from build123d import *

# Parameters (mm, degrees)
ESQUISSE1_W        = 383
ESQUISSE1_H        = 30
BOSS_EXTRU_1_DEPTH = 10
ESQUISSE2_W        = 10
ESQUISSE2_H        = 30
BOSS_EXTRU_2_DEPTH = 20
ESQUISSE3_W        = 10
ESQUISSE3_H        = 100
BOSS_EXTRU_3_DEPTH = 5


with BuildPart() as part:
    # Esquisse1 → Boss.-Extru.1 (new body)
    with BuildSketch(Plane.XY):
        Rectangle(ESQUISSE1_W, ESQUISSE1_H)
    extrude(amount=BOSS_EXTRU_1_DEPTH)

    # Esquisse2 → Boss.-Extru.2 (add)
    with BuildSketch(Plane.XY.offset(10)):
        with Locations((-186.5, 0)):
            Rectangle(ESQUISSE2_W, ESQUISSE2_H)
        with Locations((-166.5, 0)):
            Rectangle(ESQUISSE2_W, ESQUISSE2_H)
        with Locations((-146.5, 0)):
            Rectangle(ESQUISSE2_W, ESQUISSE2_H)
        with Locations((-126.5, 0)):
            Rectangle(ESQUISSE2_W, ESQUISSE2_H)
        with Locations((-106.5, 0)):
            Rectangle(ESQUISSE2_W, ESQUISSE2_H)
        with Locations((-86.5, 0)):
            Rectangle(ESQUISSE2_W, ESQUISSE2_H)
        with Locations((-66.5, 0)):
            Rectangle(ESQUISSE2_W, ESQUISSE2_H)
        with Locations((-46.5, 0)):
            Rectangle(ESQUISSE2_W, ESQUISSE2_H)
        with Locations((-26.5, 0)):
            Rectangle(ESQUISSE2_W, ESQUISSE2_H)
        with Locations((-6.5, 0)):
            Rectangle(ESQUISSE2_W, ESQUISSE2_H)
        with Locations((13.5, 0)):
            Rectangle(ESQUISSE2_W, ESQUISSE2_H)
        with Locations((33.5, 0)):
            Rectangle(ESQUISSE2_W, ESQUISSE2_H)
        with Locations((53.5, 0)):
            Rectangle(ESQUISSE2_W, ESQUISSE2_H)
        with Locations((73.5, 0)):
            Rectangle(ESQUISSE2_W, ESQUISSE2_H)
        with Locations((93.5, 0)):
            Rectangle(ESQUISSE2_W, ESQUISSE2_H)
        with Locations((113.5, 0)):
            Rectangle(ESQUISSE2_W, ESQUISSE2_H)
        with Locations((133.5, 0)):
            Rectangle(ESQUISSE2_W, ESQUISSE2_H)
        with Locations((153.5, 0)):
            Rectangle(ESQUISSE2_W, ESQUISSE2_H)
        Polygon((168.5, -15), (178.5, -15), (191.5, -15), (191.5, 15), (178.5, 15), (168.5, 15), align=None)
    extrude(amount=BOSS_EXTRU_2_DEPTH)

    # Esquisse3 → Boss.-Extru.3 (add)
    with BuildSketch(Plane.XZ.offset(15)):
        with Locations((0, -41.837008413)):
            Rectangle(ESQUISSE3_W, ESQUISSE3_H)
    extrude(amount=BOSS_EXTRU_3_DEPTH)


solid = part.part
Model file for the job. Use its own axes, mm. A direction names the side the tool comes from. Give positions to 0.01 mm unless a question says otherwise; leave off trailing zeros. Loops run counter-clockwise (first coordinate to the right, second up) from the corner with the lowest first, then second, coordinate; pieces in that order, holes last.
Item 1: Slice it at B-B (z = -7). Write the cut outline in (x, y), plus the area to 3 significant figures.
Check values:
outline: (-5, -20) - (5, -20) - (5, -15) - (-5, -15) - close
area: 50.0 mm2
Item 2: Drop flat-ended pins along their axis: P1, Ø4, axis at y = -13.5, z = -29, coming from the +X side; P2, Ø24, axis at x = -36.5, z = 20, coming from the -Y side; P3, Ø2, axis at x = -4, y = 7.5, coming from the -Z side; P4, Ø1, axis at x = -144, z = -2, coming from the +Y side. Give the stop position or say it passes through.
Check values:
P1: stops at x = 5
P2: stops at y = -15
P3: stops at z = 0
P4: passes through
Item 3: Drill centre lines: line 1 along Z through (x, y) = (-59, 4); line 2 along Z through (x, y) = (-29, -8); line 3 along X through (y, z) = (-17.5, -20). Where is each one in solid material? Low to high.
Check values:
line 1: z = 0 to 10
line 2: z = 0 to 30
line 3: x = -5 to 5
Item 4: Which spindle directions (+Z, -Z, +X, -X, +Y, -Y) get a long thin tool onto all of the face, cutting with end or side? Do faces 3 (the face through (-27, 0, 30)), 4 (the face through (-117, 0, 10)). Say none if no direction does.
Check values:
face 3: +Z, +X, -X, +Y, -Y
face 4: +Z, +Y, -Y
Item 5: Mould opens along X. For faces 1 (the face through (-167, 0, 30)), 2 (the face through (8.5, 0, 20)) say: +X half, -X half, draft (parallel to the pull), parting line (faces both ways), or undercut.
Check values:
face 1: draft
face 2: undercut
Item 6: Slice it at A-A (x = 64). Write the cut outline in (y, z).
Check values:
outline: (-15, 0) - (15, 0) - (15, 10) - (-15, 10) - close
